Could you check a few things on this model? Use its own coordinates, in mm. A direction names the side the tool comes from. Give positions to 0.01 mm unless a question says otherwise; leave off trailing zeros. Order: outer loops, then holes, each group sorted by start corner. A loop starts at its lowest first (then second) coordinate and runs counter-clockwise, first axis right, second up.
Autodesk Fusion 360 part; units mm, degrees
sketch "antenna_nupsi" plane through (0, 0, 0) normal (0, 0, 1) x (1, 0, 0)
  line L0 (0, 0) -> (0.625, 0)
  line L1 (0.625, 0) -> (1.425, 0)
  line L2 (1.425, 0) -> (6.425, 0)
  line L3 (6.425, 0) -> (7.225, 0)
  line L4 (0, 0) -> (-0.625, 0)
  line L5 (-0.625, 0) -> (-1.425, 0)
  arc A0 (2.9, 4.325) -> (-1.425, 0) centre (2.9, 0) ccw
  line L6 (1.425, 0.8) -> (1.425, 3)
  line L7 (1.425, 3) -> (6.425, 3)
  line L8 (6.425, 3) -> (6.425, 0.8)
  line L9 (2.9, 4.325) -> (6.225, 4.325)
  line L10 (7.225, 0) -> (7.225, 3.325)
  line L11 (1.425, 0.8) -> (6.425, 0.8)
  arc A1 (0.625, 0) -> (-0.625, 0) centre (0, 0) ccw
  arc A2 (1, 0) -> (-1, 0) centre (0, 0) ccw
  arc A3 (7.225, 3.325) -> (6.225, 4.325) centre (6.225, 3.325) ccw
  dimension "d1" = 1.25
  dimension "d2" = 0.8
  dimension "d5" = 0.8
  dimension "d7" = 0.8
  dimension "d8" = 2.2
  dimension "d19" = 2
  dimension "d20" = 5
extrude "Extrude5" add sketch "antenna_nupsi" along normal blind 11 contours L1 L2 L3 L5 A0 L9 L10 A2 A3 makes body 1
extrude "Extrude6" add sketch "antenna_nupsi" along normal blind 0.8 separate body contours L1 L2 L3 L5 A0 L9 L10 A2 A3 | L6 L7 L8 L11 makes body 2
move_body "Move1" bodies 2 to x (1, 0, 0) y (0, 1, 0) z (0, 0, 1) at (0, 0, 11)
combine "Combine2" operation add target body 1 tool bodies 2
chamfer "Chamfer2" distance 0.25 angle 45 4 edges at (1.425, 1.9, 0) (3.925, 0.8, 0) (6.425, 1.9, 0) (3.925, 3, 0) on bodies 1
Item 1: For pin 1 (1.5 mm diameter, centred on x = 0, z = 10.5, fed in from -Y); pin 2 (2.5 mm diameter, centred on y = 2, z = 6, fed in from -X); pin 3 (1.5 mm diameter, centred on x = 5.5, y = 2, fed in from -Z), each with a flat end and sliding along its axis, tell me the tip position at first contact or that it passes through.
Findings:
pin 1: stops at y = 0.66
pin 2: stops at x = -1.36
pin 3: stops at z = 11
Item 2: We'd pull the mould along Y, two halves only. Please class faces 1 (the flat face through (4, 0.8, 6)), 2 (the flat face through (4, 0, 6)), 3 (the flat face through (7.225, 2, 6)): +Y half, -Y half, draft (parallel to the pull), parting line (faces both ways), or undercut.
Findings:
face 1: undercut
face 2: -Y half
face 3: draft
Item 3: Imagine slicing it at D-D on x = 0.75. List the corners of the cut face in (y, z) for me, then the cut area to 3 significant figures.
Findings:
outline: (0.66, 0) - (3.75, 0) - (3.75, 11.8) - (0.66, 11.8) - close
area: 36.5 mm2
Item 4: For faces 4 (the flat face through (6.425, 2, 6)), 5 (the flat face through (4, 2, 11.8)), which set-ups out of +Z, -Z, +X, -X, +Y, -Y let a thin tool reach every point of the face, with its end or its side?
Findings:
face 4: -Z
face 5: +Z, +X, -X, +Y, -Y
Item 5: Imagine slicing it at A-A on z = 4.5. List the corners of the cut face in (x, y) for me (3 decimals).
Findings:
outline: (-1.425, 0) - (-1, 0) arc R1 cw to (1, 0) - (7.225, 0) - (7.225, 3.325) arc R1 ccw to (6.225, 4.325) - (2.9, 4.325) arc R4.325 ccw to start; hole (1.425, 0.8) - (6.425, 0.8) - (6.425, 3) - (1.425, 3) - close
Item 6: Please list where these lines run through material, in increasing order: line 1 along Y through (x, z) = (6, 6) (3 decimals); line 2 along Z through (x, y) = (5, 0.95); line 3 along X through (y, z) = (2.7, 10.75) (3 decimals).
Findings:
line 1: y = 0 to 0.8, 3 to 4.325
line 2: z = 11 to 11.8
line 3: x = -0.479 to 1.425, 6.425 to 7.225
Item 7: Imagine slicing it at C-C on y = 2.1. List the corners of the cut face in (x, z) for me (3 decimals).
Findings:
outline: (-0.881, 0) - (1.175, 0) - (1.425, 0.25) - (1.425, 11) - (6.425, 11) - (6.425, 0.25) - (6.675, 0) - (7.225, 0) - (7.225, 11.8) - (-0.881, 11.8) - close
Item 8: Imagine slicing it at B-B on x = 5.75. List the corners of the cut face in (y, z) for me (3 decimals).
Findings:
outline: (0, 0) - (0.55, 0) - (0.8, 0.25) - (0.8, 11) - (3, 11) - (3, 0.25) - (3.25, 0) - (4.325, 0) - (4.325, 11.8) - (0, 11.8) - close
